```python
from build123d import *

# Parameters (mm, degrees)
F1_DEPTH    = 76.2
F2_R        = 2.54
F3_R        = 1.27
F4_T1_DEPTH = 102.1482316142
F5_DEPTH    = 69.85


# Not quite as in the source:
# - a fillet or chamfer that OpenCascade refuses, or shapes differently, is made with other operations: its cross-section is extruded or revolved along the edge and cut away or added


with BuildPart() as f1:
    # F0 (on Front) → F1 (new body)
    with BuildSketch(Plane.XZ):
        with BuildLine():
            Line((-38.6677846295, 20.0523413639), (-43.4175846295, 20.0523413639))
            Line((-43.4175846295, 20.0523413639), (-48.3946166933, -4.8552709632))
            Line((-48.3946166933, -4.8552709632), (53.2053833067, -4.8552709632))
            ThreePointArc((53.2053833067, -4.8552709632), (23.2548005589, 18.7290020933), (-14.1116172914, 26.2792444457))
            Line((-14.1116172914, 26.2792444457), (-18.739449567, 3.119206343))
            Line((-18.739449567, 3.119206343), (-41.1563006614, 7.5985352004))
            Line((-41.1563006614, 7.5985352004), (-38.6677846295, 20.0523413639))
        make_face()
        Polygon((-41.6217533096, 3.9728981134), (-18.1607622718, -0.7150704927), (-42.558501873, -0.7150704927), align=None, mode=Mode.SUBTRACT)
        with BuildLine():
            ThreePointArc((-10.9155429452, 22.4410306257), (19.1784355797, 16.2823947845), (44.5942434068, -0.9690704107))
            Line((44.5942434068, -0.9690704107), (-15.5933427256, -0.9690704107))
            Line((-15.5933427256, -0.9690704107), (-10.9155429452, 22.4410306257))
        make_face(mode=Mode.SUBTRACT)
    extrude(amount=F1_DEPTH)

    # F2
    f2_edges = [f1.edges().sort_by_distance(p)[0] for p in [
        (-10.915543, -38.1, 22.441031),
        (-15.593343, -38.1, -0.96907),
    ]]
    fillet(f2_edges, radius=F2_R)

    # F3
    f3_edges = [f1.edges().sort_by_distance(p)[0] for p in [
        (-41.621753, -38.1, 3.972898),
        (-42.558502, -38.1, -0.71507),
    ]]
    fillet(f3_edges, radius=F3_R)

    # F4: fillet of radius 6.35 on 1 edges, made by hand

    # F4_s2 → F4_t1 (cut)
    with BuildSketch(Plane.XZ.offset(-12.9741158071)):
        with BuildLine():
            ThreePointArc((-38.6677846295, 20.0523413639), (-42.4092351432, 18.4801883775), (-44.4344758164, 14.9632981071))
            Line((-44.4344758164, 14.9632981071), (-43.4175846295, 20.0523413639))
            Line((-43.4175846295, 20.0523413639), (-38.6677846295, 20.0523413639))
        make_face()
    extrude(amount=F4_T1_DEPTH, mode=Mode.SUBTRACT)

    # F5 (cut): a face of the model
    f5_faces = [f1.faces().sort_by_distance(p)[0] for p in [
        (-45.3723710361, -76.2, 4.845766414),
    ]]
    extrude(f5_faces, amount=-F5_DEPTH, mode=Mode.SUBTRACT)


solid = f1.part
```
Input: part model. Units: mm. Frame: model coordinates. A direction names the side the tool comes from. Coordinates: 2 decimals unless noted, no trailing zeros. Loops run counter-clockwise (first coordinate to the right, second up) from the corner with the lowest first, then second, coordinate; pieces in that order, holes last. Notation, with made-up numbers: (-36, -22.75) -> (-24, -22.75) arc R3 ccw to (-24, -17.75) -> close; hole circle Ø1 at (-30.75, -31.75). An arc over 180 degrees is marked (long way). Use a Markdown table: item, result.
1) Cut plane D-D (z = 18). Return the cut outline in (x, y).
Results found:
| item | result |
|---|---|
| outline | (-42.9, -6.35) -> (-39.08, -6.35) -> (-39.08, 0) -> (-42.9, 0) -> close; (-15.77, -6.35) -> (-11.8, -6.35) -> (-11.8, 0) -> (-15.77, 0) -> close; (14.73, -6.35) -> (24.79, -6.35) -> (24.79, 0) -> (14.73, 0) -> close |
2) Material intervals for line 1 along X through (y, z) = (-5, 17); line 2 along X through (y, z) = (-6, 9); line 3 along Z through (x, y) = (29, -5.5), sorted ascending. Write a range as from..to.
Results found:
| item | result |
|---|---|
| line 1 | x = -43.64..-39.28, -15.97..-12, 17.42..26.77 |
| line 2 | x = -45.63..-40.88, -17.56..-13.6, 32.61..39.23 |
| line 3 | z = -4.86..-0.97, 11.3..15.79 |
3) Cut plane B-B (y = -2). Return the cut outline in (x, z) (3 decimals), then the cut area to 3 significant figures.
Results found:
| item | result |
|---|---|
| outline | (-48.395, -4.855) -> (53.205, -4.855) arc R82.263 ccw to (-14.112, 26.279) -> (-18.739, 3.119) -> (-41.156, 7.599) -> (-38.668, 20.052) arc R6.35 ccw to (-44.434, 14.963) -> close; hole (-42.255, 0.804) arc R1.27 ccw to (-41.01, -0.715) -> (-18.161, -0.715) -> (-40.376, 3.724) arc R1.27 ccw to (-41.871, 2.728) -> close; hole (-14.986, 2.069) arc R2.54 ccw to (-12.496, -0.969) -> (44.594, -0.969) arc R78.377 ccw to (-8.759, 22.401) arc R2.54 ccw to (-11.331, 20.36) -> close |
| area | 936 mm2 |
4) Cut plane A-A (z = 9.5). Return the cut outline in (x, y), then the cut area to 3 significant figures.
Results found:
| item | result |
|---|---|
| outline | (-45.53, -6.35) -> (-40.78, -6.35) -> (-40.78, 0) -> (-45.53, 0) -> close; (-17.46, -6.35) -> (-13.5, -6.35) -> (-13.5, 0) -> (-17.46, 0) -> close; (31.86, -6.35) -> (38.58, -6.35) -> (38.58, 0) -> (31.86, 0) -> close |
| area | 98.0 mm2 |
5) Cut plane C-C (x = 28.5). Return the cut outline in (y, z).
Results found:
| item | result |
|---|---|
| outline | (-6.35, -4.86) -> (0, -4.86) -> (0, -0.97) -> (-6.35, -0.97) -> close; (-6.35, 11.6) -> (0, 11.6) -> (0, 16.07) -> (-6.35, 16.07) -> close |
6) Contact query for a flat-ended pin moving along its axis: pin 1 (3 mm diameter, centred on x = -27, y = -4.5, fed in from +Z). Output: stop coordinate, or through.
Results found:
| item | result |
|---|---|
| pin 1 | stops at z = 5.07 |
7) Access query for faces 1 (the flat face through (-16.393, -3.131, 14.861)), 2 (the flat face through (2, -3, -4.855)), 3 (the flat face through (-39.93, -3.13, 13.74)). Directions: +Z, -Z, +X, -X, +Y, -Y. A direction counts if a zero-diameter tool reaches every point of the face in a straight line with its end or side. Return the directions, or none.
Results found:
| item | result |
|---|---|
| face 1 | +Z, +Y, -Y |
| face 2 | -Z, +X, -X, +Y, -Y |
| face 3 | +Y, -Y |
8) Pull-direction query (X, two-part tool) for faces 4 (the flat face through (-42.065, -3.131, 1.752)), 5 (the flat face through (-46.387, -3.131, 5.193)), 6 (the flat face through (-5, -6.35, -3)); classes: released by +X, released by -X, zero draft, split by the parting line, or undercut.
Results found:
| item | result |
|---|---|
| face 4 | undercut |
| face 5 | released by -X |
| face 6 | zero draft |
